Geometry check sheet. Reference: the model listing, model coordinates, mm. Face numbers are marked on the shaded views. A direction names the side the tool comes from. Round coordinates to 2 decimals unless told otherwise and drop trailing zeros. Loops run counter-clockwise (first coordinate to the right, second up) from the corner with the lowest first, then second, coordinate; pieces in that order, holes last. Notation, with made-up numbers: M -39,61.25 L 18,61.25 A8 ccw 18,69.25 Z; hole C -15.75,1 d6. An arc over 180 degrees is marked long. Write item = value, one per line.
from build123d import *

# Parameters (mm, degrees)
F2_SIZE = 0.5


with BuildPart() as f1:
    # F0 (on Right) → F1 (revolve)
    with BuildSketch(Plane.YZ):
        Polygon((4.5, 8), (0, 8), (0, 4.5), (11.5, 4.5), (11.5, 10), (4.5, 10), align=None)
    revolve(axis=Axis((0, 13.707888, 0), (0, 1, 0)))

    # F2
    f2_edges = [f1.edges().sort_by_distance(p)[0] for p in [
        (0, 11.5, -4.5),
        (0, 0, -4.5),
        (0, 4.5, -10),
        (0, 11.5, -10),
        (0, 0, -8),
    ]]
    chamfer(f2_edges, length=F2_SIZE)


solid = f1.part
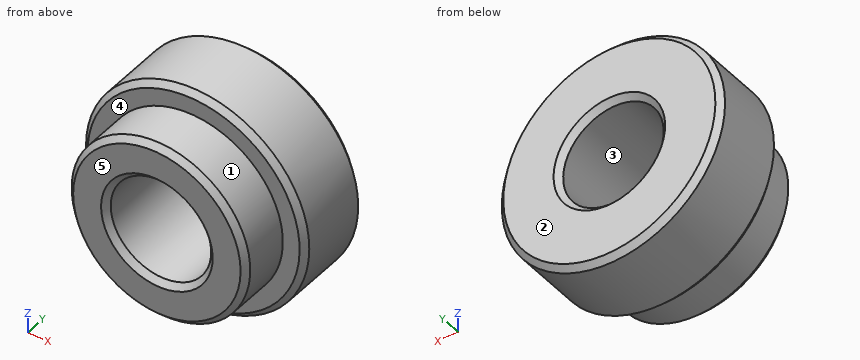
(1) Sectioned sample at C-C on y = 9.25. Record the cut outline in (x, z).
Result set:
outline = C 0,0 d20; hole C 0,0 d9
(2) Material ranges on line 1 along X through (y, z) = (3.75, 0); line 2 along Z through (x, y) = (3, 6.5); line 3 along X through (y, z) = (10, -3.5), recorded low to high. Write a range as from..to.
Result set:
line_1 = -8..-4.5, 4.5..8
line_2 = -9.54..-3.35, 3.35..9.54
line_3 = -9.37..-2.83, 2.83..9.37
(3) Sectioned sample at D-D on y = 2. Record the cut outline in (x, z), then the cut area to 3 significant figures.
Result set:
outline = C 0,0 d16; hole C 0,0 d9
area = 137 mm2
(4) Tool access check on the marked faces 4 and 5. Record the directions out of +Z, -Z, +X, -X, +Y, -Y that give a thin tool (end or side, any length) a straight path to the whole face; none if there is none.
Result set:
face_4 = -Y
face_5 = +Z, -Z, +X, -X, -Y
(5) Depth check by flat-ended pin: pin 1 Ø10 at (x, z) = (1.5, -2.5) entering from +Y; pin 2 Ø1 at (y, z) = (6.5, -2.5) entering from -X; pin 3 Ø1.5 at (x, z) = (3.5, 1.5) entering from +Y; pin 4 Ø1.5 at (x, z) = (5.5, 8) entering from -Y. Enter the tip coordinate at first touch or a pass-through.
Result set:
pin_1 = 11.5
pin_2 = -9.8
pin_3 = 11.06
pin_4 = 4.5
(6) Sectioned sample at B-B on x = 0. Record the cut outline in (y, z), then the cut area to 3 significant figures.
Result set:
outline = M 0,-7.5 L 0.5,-8 L 4.5,-8 L 4.5,-9.5 L 5,-10 L 11,-10 L 11.5,-9.5 L 11.5,-5 L 11,-4.5 L 0.5,-4.5 L 0,-5 Z; M 0,5 L 0.5,4.5 L 11,4.5 L 11.5,5 L 11.5,9.5 L 11,10 L 5,10 L 4.5,9.5 L 4.5,8 L 0.5,8 L 0,7.5 Z
area = 107 mm2
(7) Sectioned sample at A-A on z = 0. Record the cut outline in (x, y).
Result set:
outline = M -10,5 L -9.5,4.5 L -8,4.5 L -8,0.5 L -7.5,0 L -5,0 L -4.5,0.5 L -4.5,11 L -5,11.5 L -9.5,11.5 L -10,11 Z; M 4.5,0.5 L 5,0 L 7.5,0 L 8,0.5 L 8,4.5 L 9.5,4.5 L 10,5 L 10,11 L 9.5,11.5 L 5,11.5 L 4.5,11 Z
(8) Release check for a two-part mould opening along Z. For the marked faces 1, 2 and 3 record: released by +Z, released by -Z, zero draft, split by the parting line, or undercut.
Result set:
face_1 = split by the parting line
face_2 = zero draft
face_3 = undercut
